Check sheet for the modelled part. Datum: model origin and axes. Units: mm. Face numbers are marked on the shaded views. A direction names the side the tool comes from. Round coordinates to 2 decimals unless told otherwise and drop trailing zeros. Loops run counter-clockwise (first coordinate to the right, second up) from the corner with the lowest first, then second, coordinate; pieces in that order, holes last. Notation, with made-up numbers: (61.5, 69) - (99.5, 69) arc R20 ccw to (99.5, 108) - close; hole circle Ø4 at (41, 5.5). An arc over 180 degrees is marked (long way). Answer in a Markdown table with one row per item. Add a question column.
(1) Cross-section at C-C on x = -7. Enter the section's corners in (y, z), then the cut area to 3 significant figures.
(2) Access from +Z, -Z, +X, -X, +Y, -Y to the whole of each face (thin tool, end or side, straight path). Record for the marked faces 1, 2 and 3.
(3) Gauge pin test, flat ends, axial feed: pin 1 (4 mm diameter, centred on y = -1, z = -2.5, fed in from -X); pin 2 (6 mm diameter, centred on x = 0, z = -13, fed in from -Y); pin 3 (1 mm diameter, centred on y = -3.5, z = -3, fed in from +X); pin 4 (1 mm diameter, centred on y = -8, z = -2, fed in from +X). Record the tip position at first contact, or that the pin passes through.
(4) Mould release check, pull along Y, two halves, no side actions. Record for the marked faces 4, 5 and 6: +Y half, -Y half, draft (parallel to the pull), parting line (faces both ways), or undercut.
(5) Cross-section at D-D on z = -4.25. Enter the section's corners in (x, y), then the cut area to 3 significant figures.
(6) Thickness scan on line 1 along Y through (x, z) = (0, -3.2); line 2 along Y through (x, z) = (0, -10.5); line 3 along Z through (x, y) = (-5.5, -4.5). Record the ranges inside material, lowest first.
(7) Cross-section at A-A on x = 0. Enter the section's corners in (y, z).
(8) Cross-section at B-B on y = -1.25. Enter the section's corners in (x, z).
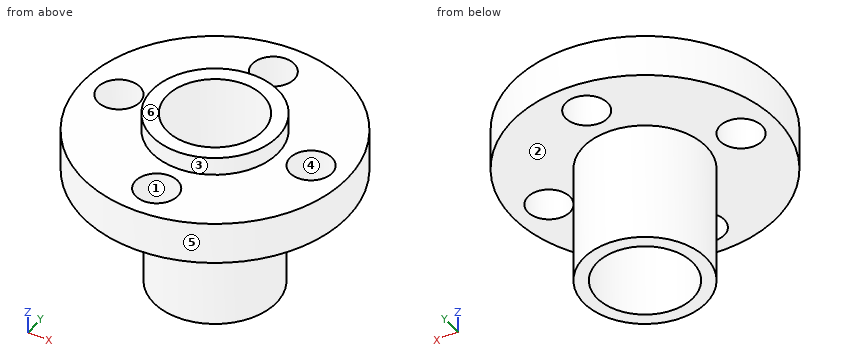
from build123d import *

# Parameters (mm, degrees)
SKETCH1_R           = 5.25
BOSS_EXTRUDE1_DEPTH = 1.5
SKETCH2_R           = 11
BOSS_EXTRUDE2_DEPTH = 3.5
SKETCH3_R           = 5.1
BOSS_EXTRUDE3_DEPTH = 10
SKETCH4_R           = 4
CUT_EXTRUDE1_DEPTH  = 22.610182785
SKETCH5_R           = 1.75
CUT_EXTRUDE2_DEPTH  = 10


with BuildPart() as part:
    # Sketch1 → Boss-Extrude1 (new body)
    with BuildSketch(Plane.XY):
        Circle(SKETCH1_R)
    extrude(amount=-BOSS_EXTRUDE1_DEPTH)

    # Sketch2 → Boss-Extrude2 (add)
    with BuildSketch(Plane(origin=(0, 0, -1.5), x_dir=(-1, 0, 0), z_dir=(0, 0, -1))):
        Circle(SKETCH2_R)
    extrude(amount=BOSS_EXTRUDE2_DEPTH)

    # Sketch3 → Boss-Extrude3 (add)
    with BuildSketch(Plane(origin=(0, 0, -5), x_dir=(-1, 0, 0), z_dir=(0, 0, -1))):
        Circle(SKETCH3_R)
    extrude(amount=BOSS_EXTRUDE3_DEPTH)

    # Sketch4 → Cut-Extrude1 (cut, through all)
    with BuildSketch(Plane(origin=(0, 0, -15), x_dir=(-1, 0, 0), z_dir=(0, 0, -1))):
        Circle(SKETCH4_R)
    extrude(amount=-CUT_EXTRUDE1_DEPTH, mode=Mode.SUBTRACT)

    # Sketch5 → Cut-Extrude2 (cut)
    with BuildSketch(Plane.XY.offset(-1.5)):
        with Locations((-8, 0)):
            Circle(SKETCH5_R)
        with Locations((0, 8)):
            Circle(SKETCH5_R)
        with Locations((8, 0)):
            Circle(SKETCH5_R)
        with Locations((0, -8)):
            Circle(SKETCH5_R)
    extrude(amount=-CUT_EXTRUDE2_DEPTH, mode=Mode.SUBTRACT)


solid = part.part
Answers:
| question | item | result |
|---|---|---|
| 1 | outline | (-8.49, -5) - (-1.44, -5) - (-1.44, -1.5) - (-8.49, -1.5) - close; (1.44, -5) - (8.49, -5) - (8.49, -1.5) - (1.44, -1.5) - close |
| 1 | area | 49.3 mm^2 |
| 2 | face 1 | +Z, -Z |
| 2 | face 2 | -Z |
| 2 | face 3 | +Z |
| 3 | pin 1 | stops at x = -11 |
| 3 | pin 2 | stops at y = -5.1 |
| 3 | pin 3 | stops at x = 10.58 |
| 3 | pin 4 | stops at x = 8.05 |
| 4 | face 4 | undercut |
| 4 | face 5 | parting line |
| 4 | face 6 | draft |
| 5 | outline | circle Ø22 at (0, 0); hole circle Ø3.5 at (-8, 0); hole circle Ø8 at (0, 0); hole circle Ø3.5 at (0, -8); hole circle Ø3.5 at (0, 8); hole circle Ø3.5 at (8, 0) |
| 5 | area | 291 mm^2 |
| 6 | line 1 | y = -11 to -9.75, -6.25 to -4, 4 to 6.25, 9.75 to 11 |
| 6 | line 2 | y = -5.1 to -4, 4 to 5.1 |
| 6 | line 3 | z = -5 to -1.5 |
| 7 | outline | (-11, -5) - (-9.75, -5) - (-9.75, -1.5) - (-11, -1.5) - close; (-6.25, -5) - (-5.1, -5) - (-5.1, -15) - (-4, -15) - (-4, 0) - (-5.25, 0) - (-5.25, -1.5) - (-6.25, -1.5) - close; (4, -15) - (5.1, -15) - (5.1, -5) - (6.25, -5) - (6.25, -1.5) - (5.25, -1.5) - (5.25, 0) - (4, 0) - close; (9.75, -5) - (11, -5) - (11, -1.5) - (9.75, -1.5) - close |
| 8 | outline | (-10.93, -5) - (-9.22, -5) - (-9.22, -1.5) - (-10.93, -1.5) - close; (-6.78, -5) - (-4.94, -5) - (-4.94, -15) - (-3.8, -15) - (-3.8, 0) - (-5.1, 0) - (-5.1, -1.5) - (-6.78, -1.5) - close; (3.8, -15) - (4.94, -15) - (4.94, -5) - (6.78, -5) - (6.78, -1.5) - (5.1, -1.5) - (5.1, 0) - (3.8, 0) - close; (9.22, -5) - (10.93, -5) - (10.93, -1.5) - (9.22, -1.5) - close |
